Build history of the part. All positions in model axes, mm. A direction names the side the tool comes from. Coordinates: 2 decimals unless noted, no trailing zeros. Order: outer loops, then holes, each group sorted by start corner. A loop starts at its lowest first (then second) coordinate and runs counter-clockwise, first axis right, second up. Notation, with made-up numbers: M -7,-0.75 L 35,-0.75 A6 cw 35,9.25 Z; hole C -30.5,69.5 d6. An arc over 180 degrees is marked long. Write item = value, one per line. Start each with the question number.
Q1. Pin check, flat tips, straight feed: P1, Ø2.5, axis at x = 92, z = -5, coming from the -Y side; P2, Ø18, axis at x = 60.5, z = 38, coming from the +Y side. Stop position of each tip, or through.
Q2. Drill centre lines: probe 1 along X at (y, z) = (3.5, 65); probe 2 along Z at (x, y) = (-5, 4.75); probe 3 along X at (y, z) = (9.25, 16). Where is each one in solid material? Low to high.
Q3. Pull direction Y, two halves, no side cores. Call faces 4 (the face through (43, 10, 65)), 5 (the face through (13, 9.753, -5)), 6 (the face through (14, 4.753, -5)), 7 (the face through (-6.45, 4.93, -4.94)): released by +Y, released by -Y, zero draft, split by the parting line, or undercut.
Q4. Band-saw the part on A-A on z = 65. Write the cut outline in (x, y), plus the area to 3 significant figures.
Q5. Band-saw the part on B-B on x = -5. Write the cut outline in (y, z), plus the area to 3 significant figures.
Q6. Band-saw the part on D-D on y = 6.5. Write the cut outline in (x, z).
Q7. Band-saw the part on C-C on z = -5. Write the cut outline in (x, y), plus the area to 3 significant figures.
Q8. 3-axis set-ups, long thin cutter, end or side, ignore diameter. For faces 1 (the face through (8.527, 7, -5)), 2 (the face through (44, 6, 60)), 3 (the face through (-10, 5, 31)): which of +Z, -Z, +X, -X, +Y, -Y reach the whole face in a straight line?
Autodesk Fusion 360 part; units mm, degrees
sketch "Sketch1" plane through (0, 0, 0) normal (0, 1, 0) x (1, 0, 0)
  line L0 (0, 0) -> (87, 0)
  line L1 (87, 0) -> (87, -60)
  line L2 (87, -60) -> (0, -60)
  line L3 (0, -60) -> (0, 0)
  line L4 (-10, 10) -> (97, 10)
  line L5 (97, 10) -> (97, -70)
  line L6 (97, -70) -> (-10, -70)
  line L7 (-10, -70) -> (-10, 10)
  circle A0 centre (-5, 5) radius 1.45
  circle A1 centre (-5, -65) radius 1.45
  circle A2 centre (92, -65) radius 1.45
  circle A3 centre (92, 5) radius 1.45
  dimension "d1" = 87
  dimension "d2" = 60
  dimension "d3" = 107
  dimension "d4" = 80
  dimension "d5" = 10
  dimension "d6" = 2.9
  dimension "d7" = 5
  dimension "d8" = 2.9
  dimension "d9" = 5
  dimension "d10" = 5
  dimension "d11" = 2.9
  dimension "d12" = 5
  dimension "d13" = 5
  dimension "d14" = 2.9
  dimension "d15" = 5
  dimension "d16" = 5
extrude "Extrude1" add sketch "Sketch1" along normal blind 3 contours L0 L1 L2 L3 | L4 L5 L6 L7
extrude "Extrude2" cut sketch "Sketch1" along normal blind 10
extrude "Extrude3" add sketch "Sketch1" along normal blind 10
sketch "Sketch3" plane through (0, 0, 0) normal (0, 0, 1) x (1, 0, 0)
  line L0 (8.5266, 9.753) -> (18.5266, 9.753)
  line L1 (18.5266, 9.753) -> (18.5266, 4.753)
  line L2 (18.5266, 4.753) -> (8.5266, 4.753)
  line L3 (8.5266, 4.753) -> (8.5266, 9.753)
  dimension "d23" = 10
  dimension "d24" = 5
extrude "Extrude4" cut sketch "Sketch3" against normal blind 10
Recorded:
q1.P1 = through
q1.P2 = 3
q2.probe_1 = -10 to -6.45, -3.55 to 90.55, 93.45 to 97
q2.probe_2 = -10 to -6.45, -3.55 to 63.55, 66.45 to 70
q2.probe_3 = -10 to 0, 87 to 97
q3.face_4 = released by +Y
q3.face_5 = undercut
q3.face_6 = undercut
q3.face_7 = zero draft
q4.outline = M -10,0 L -6.45,0 L -6.45,10 L -10,10 Z; M -3.55,0 L 90.55,0 L 90.55,10 L -3.55,10 Z; M 93.45,0 L 97,0 L 97,10 L 93.45,10 Z
q4.area = 1,010 mm2
q5.outline = M 0,-10 L 10,-10 L 10,-6.45 L 0,-6.45 Z; M 0,-3.55 L 10,-3.55 L 10,63.55 L 0,63.55 Z; M 0,66.45 L 10,66.45 L 10,70 L 0,70 Z
q5.area = 742 mm2
q6.outline = M -10,-10 L 8.53,-10 L 8.53,0 L 0,0 L 0,60 L 87,60 L 87,0 L 18.53,0 L 18.53,-10 L 97,-10 L 97,70 L -10,70 Z; hole C -5,-5 d2.9; hole C -5,65 d2.9; hole C 92,-5 d2.9; hole C 92,65 d2.9
q7.outline = M -10,0 L -6.45,0 L -6.45,10 L -10,10 Z; M -3.55,0 L 90.55,0 L 90.55,10 L -3.55,10 Z; M 93.45,0 L 97,0 L 97,10 L 93.45,10 Z; hole M 8.53,4.75 L 18.53,4.75 L 18.53,9.75 L 8.53,9.75 Z
q7.area = 962 mm2
q8.face_1 = -Z
q8.face_2 = +Y
q8.face_3 = +Z, -Z, -X, +Y, -Y
